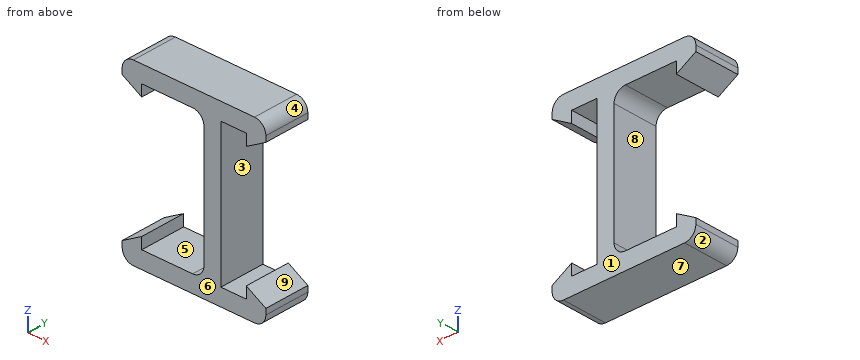
Autodesk Inventor part; units mm, degrees
ref_plane "Work Plane1" through (4.5359, -20, 3) normal (-1, 0, 0) x (0, 0, 1)
ref_plane "Work Plane2" through (-9.4641, -20, 3) normal (-1, 0, 0) x (0, 0, 1)
ref_plane "YZ Plane" through (0, 0, 0) normal (1, 0, 0) x (0, 1, 0)
sketch "Sketch1" plane through (0, 0, 0) normal (0, 0, 1) x (1, 0, 0)
  line L0 (-12.5, -12) -> (12.5, -12)
  line L1 (12.5, -12) -> (12.5, -20)
  line L2 (12.5, -20) -> (-12.5, -20)
  line L3 (-12.5, -20) -> (-12.5, -12)
  point P0 (0, 0)
  dimension "d0" = 25
  dimension "d1" = 8
  dimension "d2" = 12.5
  dimension "d3" = 20
extrude "Extrusion1" add sketch "Sketch1" along normal blind 3
sketch "Sketch3" plane through (-12.5, -20, 0) normal (0, -1, 0) x (1, 0, 0)
  line L0 (25, 3) -> (0, 3)
  line L1 (25, 0) -> (25, 3)
  line L2 (21.5359, 3) -> (21.5359, 5)
  line L3 (25, 3) -> (21.5359, 3)
  line L4 (25, 0) -> (0, 0)
  line L5 (21.5359, 5) -> (25, 3)
  point P0 (12.5, 0)
  dimension "d9" = 2
  dimension "d11" = 0
  dimension "d15" = 30
extrude "Extrusion2" add sketch "Sketch3" against normal blind 8
ref_plane "Work Plane1" through (4.5359, -20, 3) normal (-1, 0, 0) x (0, 0, 1)
sketch "Sketch4" plane through (4.5359, -20, 3) normal (-1, 0, 0) x (0, 0, 1)
  line L0 (0, 8) -> (12.5, 8)
  line L1 (12.5, 8) -> (12.5, 0)
  line L2 (12.5, 0) -> (0, 0)
  line L3 (0, 0) -> (0, 8)
  point P0 (-3, 20)
  dimension "d16" = 12.5
  dimension "d17" = 8
  dimension "d18" = 12
  dimension "d19" = 3
extrude "Extrusion3" add sketch "Sketch4" along normal blind 3
ref_plane "Work Plane2" through (-9.4641, -20, 3) normal (-1, 0, 0) x (0, 0, 1)
sketch "Sketch5" plane through (-12.5, -20, 0) normal (0, -1, 0) x (1, 0, 0)
  line L0 (21.5359, 3) -> (17.0359, 3)
  line L1 (17.0359, 15.5) -> (17.0359, 3)
  line L2 (17.0359, 15.5) -> (14.0359, 15.5)
  line L3 (14.0359, 15.5) -> (14.0359, 3)
  line L4 (14.0359, 3) -> (0, 3)
  line L5 (0, 0) -> (0, 3)
  line L6 (25, 0) -> (0, 0)
  line L7 (25, 0) -> (25, 3)
  line L8 (21.5359, 5) -> (25, 3)
  line L9 (21.5359, 3) -> (21.5359, 5)
  line L10 (3.018, 3) -> (3.018, 5)
  line L11 (3.018, 5) -> (-0.4461, 3)
  line L12 (-0.4461, 3) -> (3.018, 3)
  line L13 (-0.4461, 3) -> (0, 3)
  line L14 (0, 3) -> (0, 0)
  line L15 (0, 0) -> (-0.4461, 0)
  line L16 (-0.4461, 0) -> (-0.4461, 3)
  point P0 (12.5, 0)
  dimension "d23" = 2
  dimension "d24" = 60
extrude "Extrusion4" add sketch "Sketch5" against normal blind 8
mirror "Mirror1" about plane through (4.5359, -12, 15.5) normal (0, 0, 1) of "Extrusion1", "Extrusion2", "Extrusion3", "Extrusion4"
fillet "Fillet1" radius 2 2 edges at (1.5359, -16, 28) (1.5359, -16, 3)
fillet "Fillet2" radius 2 4 edges at (-12.9461, -16, 31) (-12.9461, -16, 0) (12.5, -16, 31) (12.5, -16, 0)
ref_plane "Work Plane3" through (4.5359, -20, 28) normal (1, 0, 0) x (0, 0, -1)
ref_plane "Work Plane4" through (-9.4641, -20, 28) normal (1, 0, 0) x (0, 0, -1)
properties part number "claw"
The model under review builds one solid part; all positions refer to its coordinate system, in mm. Face numbers are marked on the shaded views. A direction names the side the tool comes from. Round coordinates to 2 decimals unless told otherwise and drop trailing zeros. Loops run counter-clockwise (first coordinate to the right, second up) from the corner with the lowest first, then second, coordinate; pieces in that order, holes last. Notation, with made-up numbers: M 43.25,29 L 81.25,29 A25 ccw 81.25,41 Z; hole C 12,-8 d10. An arc over 180 degrees is marked long. Answer as a JSON object with one key per item and string values.
Item 1: Clearance check with flat-ended pins moving along their axes: P1, Ø1, axis at y = -18, z = 5, coming from the -X side; P2, Ø1.5, axis at y = -18, z = 19, coming from the +X side; P3, Ø1.5, axis at y = -17, z = 27, coming from the -X side; P4, Ø12, axis at x = -6, z = 17, coming from the +Y side. State where each tip first meets the part, or that it passes through.
Check sheet entries:
{"P1": "x = -10.35", "P2": "x = 4.54", "P3": "x = -12.51", "P4": "through"}
Item 2: We need section B-B, the plane y = -18.75. State the section outline as (x, z) points.
Check sheet entries:
{"outline": "M -12.95,2 A2 ccw -10.95,0 L 10.5,0 A2 ccw 12.5,2 L 12.5,3 L 9.04,5 L 9.04,3 L 4.54,3 L 4.54,28 L 9.04,28 L 9.04,26 L 12.5,28 L 12.5,29 A2 ccw 10.5,31 L -10.95,31 A2 ccw -12.95,29 L -12.95,28 L -9.48,26 L -9.48,28 L -0.46,28 A2 cw 1.54,26 L 1.54,5 A2 cw -0.46,3 L -9.48,3 L -9.48,5 L -12.95,3 Z"}
Item 3: We need section C-C, the plane z = 16. State the section outline as (x, y) points.
Check sheet entries:
{"outline": "M 1.54,-20 L 4.54,-20 L 4.54,-12 L 1.54,-12 Z"}
Item 4: Tool access review of the marked faces 5, 6, 7, 8 and 9: name each direction out of +Z, -Z, +X, -X, +Y, -Y from which nothing blocks a thin tool from reaching the whole face with its end or side.
Check sheet entries:
{"face 5": "+Y, -Y", "face 6": "+Z, -Z, +X, -X, -Y", "face 7": "-Z, +X, -X, +Y, -Y", "face 8": "-X, +Y, -Y", "face 9": "+X, +Y, -Y"}
Item 5: We need section A-A, the plane x = 7.75. State the section outline as (y, z) points, and give its area (3 significant figures).
Check sheet entries:
{"outline": "M -20,0 L -12,0 L -12,3 L -20,3 Z; M -20,28 L -12,28 L -12,31 L -20,31 Z", "area": "48.0 mm2"}
Item 6: For line 1 along Z through (x, y) = (8.5, -15); line 2 along X through (y, z) = (-13.25, 4.5); line 3 along X through (y, z) = (-14.25, 15.5), list the stretches that pass through material, from the lowest coordinate up.
Check sheet entries:
{"line 1": "0 to 3, 28 to 31", "line 2": "-10.35 to -9.48, 1.47 to 4.54, 9.04 to 9.9", "line 3": "1.54 to 4.54"}
Item 7: The part is to be moulded in two halves that separate along Z. For the marked faces 1, 2, 3 and 4, say which applies: +Z half, -Z half, draft (parallel to the pull), parting line (faces both ways), or undercut.
Check sheet entries:
{"face 1": "draft", "face 2": "-Z half", "face 3": "undercut", "face 4": "+Z half"}
